from build123d import *

# Parameters (mm, degrees)
SKETCH1_W                           = 44
SKETCH1_H                           = 45
BASE_DEPTH                          = 5
WIRE_GROOVES_DEPTH                  = 51.338851795
SLANTED_START                       = -22
SLANTED_SCREW_PLATFORM_DEPTH        = 5
SKETCH5_R                           = 2.75
MOUNTING_HOLE_SCREW_INSERTION_DEPTH = 36.040152348
SKETCH6_W                           = 5
SKETCH6_H                           = 3
ZIP_TIE_SLOTS_DEPTH                 = 34.699235283
SKETCH7_R                           = 1.425
MOUNT_CLAMPING_HOLES_DEPTH          = 34.699235283
EDGE_FILLETS_R                      = 1


with BuildPart() as part:
    # Sketch1 → Base (new body)
    with BuildSketch(Plane.XY):
        Rectangle(SKETCH1_W, SKETCH1_H)
    extrude(amount=BASE_DEPTH)

    # Sketch2 → Wire Grooves (cut, through all)
    with BuildSketch(Plane(origin=(0, 22.5, 0), x_dir=(1, 0, 0), z_dir=(0, 1, 0))):
        with BuildLine():
            Line((12, 0), (18, 0))
            ThreePointArc((18, 0), (17.443502884, -1.343502884), (16.1, -1.9))
            Line((16.1, -1.9), (13.9, -1.9))
            ThreePointArc((13.9, -1.9), (12.556497116, -1.343502884), (12, 0))
        make_face()
        with BuildLine():
            Line((-7.7, -1.9), (-9.9, -1.9))
            ThreePointArc((-9.9, -1.9), (-11.243502884, -1.343502884), (-11.8, 0))
            Line((-11.8, 0), (-5.8, 0))
            ThreePointArc((-5.8, 0), (-6.356497116, -1.343502884), (-7.7, -1.9))
        make_face()
    extrude(amount=-WIRE_GROOVES_DEPTH, mode=Mode.SUBTRACT)

    # Sketch4 → Slanted Screw Platform (add, symmetric)
    with BuildSketch(Plane(origin=(22, 0, 0), x_dir=(0, 0, -1), z_dir=(1, 0, 0)).offset(SLANTED_START)):
        Polygon((-5, -22.5), (-5, 22.5), (-17.057713659, 22.5), align=None)
    extrude(amount=SLANTED_SCREW_PLATFORM_DEPTH, both=True)

    # Sketch5 → Mounting Hole Screw Insertion (cut, through all)
    with BuildSketch(Plane(origin=(0, -2.757214207, 10.290063509), x_dir=(1, 0, 0), z_dir=(0, -0.2588190451025216, 0.9659258262890681))):
        with Locations(Location((0, 16, 0), (0, 0, 270))):
            Circle(SKETCH5_R)
    extrude(amount=-MOUNTING_HOLE_SCREW_INSERTION_DEPTH, mode=Mode.SUBTRACT)

    # Sketch6 → Zip Tie Slots (cut, through all)
    with BuildSketch(Plane.XY.offset(5)):
        with Locations((-16, 18)):
            Rectangle(SKETCH6_W, SKETCH6_H)
        with Locations((8, 18)):
            Rectangle(SKETCH6_W, SKETCH6_H)
    extrude(amount=-ZIP_TIE_SLOTS_DEPTH, mode=Mode.SUBTRACT)

    # Sketch7 → Mount Clamping Holes (cut, through all)
    with BuildSketch(Plane.XY.offset(5)):
        with Locations((-18, -18.5)):
            Circle(SKETCH7_R)
        with Locations(Location((9, -18.5, 0), (0, 0, 180))):
            Circle(SKETCH7_R)
    extrude(amount=-MOUNT_CLAMPING_HOLES_DEPTH, mode=Mode.SUBTRACT)

    # Edge Fillets
    edge_fillets_edges = [part.edges().sort_by_distance(p)[0] for p in [
        (-22, 0, 5),
        (-13.5, 22.5, 5),
        (-5, 22.5, 11.02885683),
        (0, 22.5, 17.057713659),
        (22, 0, 5),
        (5, 22.5, 11.02885683),
        (22, -22.5, 2.5),
        (-22, -22.5, 2.5),
        (-22, 22.5, 2.5),
        (22, 22.5, 2.5),
        (13.5, 22.5, 5),
    ]]
    fillet(edge_fillets_edges, radius=EDGE_FILLETS_R)


solid = part.part
Check sheet for the modelled part. Datum: model origin and axes. Units: mm. A direction names the side the tool comes from. Give positions to 0.01 mm unless a question says otherwise; leave off trailing zeros. Loops run counter-clockwise (first coordinate to the right, second up) from the corner with the lowest first, then second, coordinate; pieces in that order, holes last. Notation, with made-up numbers: M 62,22 L 98,22 A23 ccw 98,58 Z; hole C 30,10.25 d7. An arc over 180 degrees is marked long. Use a Markdown table: item, result. Add a question column.
Q1. Sectioned sample at B-B, the plane y = -18.5. Record the cut outline in (x, z) (3 decimals), then the cut area to 3 significant figures.
Q2. Mould release check, pull along Y, two halves, no side actions. Record for faces 5 (the flat face through (-5, 5, 10)), 6 (the cylindrical face through (-12.381, 22.215, 4.699)), 7 (the flat face through (-18.5, 18, 3)), 8 (the flat face through (-16, 16.5, 3)): pulls with the +Y half, pulls with the -Y half, needs draft (parallel to the pull), parting line crosses it, or undercut.
Q3. Sectioned sample at C-C, the plane x = -2. Record the cut outline in (y, z), then the cut area to 3 significant figures.
Q4. Sectioned sample at D-D, the plane y = -6. Record the cut outline in (x, z).
Q5. Go/stop test with flat-tipped pins: pin 1 (1.1 mm diameter, centred on x = 15.5, y = -7.5, fed in from -Z); pin 2 (6 mm diameter, centred on y = 5.5, z = 13.5, fed in from +X); pin 3 (9.5 mm diameter, centred on y = 7.5, z = 11, fed in from -X); pin 4 (2.5 mm diameter, centred on x = 9, y = -18.5, fed in from +Z). Record where each tip stops, or that it passes through.
Q6. Scan lines: line 1 along Y through (x, z) = (-18, 3.4) (3 decimals); line 2 along Y through (x, z) = (9.5, 3.5); line 3 along X through (y, z) = (8, 6). Record each from-to range of solid material in increasing order. Write a range as [from, to].
Q7. Tool access check on faces 1 (the flat face through (5.5, 18, 3)), 2 (the cylindrical face through (-11.229, 0.315, 1.358)), 3 (the cylindrical face through (12.619, 22.215, 4.699)), 4 (the flat face through (-13, 0, 5)). Record the directions out of +Z, -Z, +X, -X, +Y, -Y that give a thin tool (end or side, any length) a straight path to the whole face; none if there is none.
Q8. Sectioned sample at A-A, the plane x = 9. Record the cut outline in (y, z) (3 decimals), then the cut area to 3 significant figures.
Verdict:
| question | item | result |
|---|---|---|
| 1 | outline | M -22,0 L -19.425,0 L -19.425,5 L -21,5 A1 ccw -22,4 Z; M -16.575,0 L -11.8,0 A1.9 cw -9.9,1.9 L -7.7,1.9 A1.9 cw -5.8,0 L 7.575,0 L 7.575,5 L 5,5 L 5,6.072 L -5,6.072 L -5,5 L -16.575,5 Z; M 10.425,0 L 12,0 A1.9 cw 13.9,1.9 L 16.1,1.9 A1.9 cw 18,0 L 22,0 L 22,4 A1 ccw 21,5 L 10.425,5 Z |
| 1 | area | 182 mm^2 |
| 2 | face 5 | needs draft |
| 2 | face 6 | pulls with the +Y half |
| 2 | face 7 | undercut |
| 2 | face 8 | undercut |
| 3 | outline | M -22.5,0 L 14.61,0 L 10.87,13.94 L -22.5,5 Z; M 14.52,14.92 L 18.52,0 L 22.5,0 L 22.5,15.75 A1 ccw 21.24,16.72 Z |
| 3 | area | 440 mm^2 |
| 4 | outline | M -22,0 L -11.8,0 A1.9 cw -9.9,1.9 L -7.7,1.9 A1.9 cw -5.8,0 L 12,0 A1.9 cw 13.9,1.9 L 16.1,1.9 A1.9 cw 18,0 L 22,0 L 22,4 A1 ccw 21,5 L 5,5 L 5,9.42 L -5,9.42 L -5,5 L -21,5 A1 ccw -22,4 Z |
| 5 | pin 1 | z = 1.9 |
| 5 | pin 2 | x = 5 |
| 5 | pin 3 | x = -5 |
| 5 | pin 4 | through |
| 6 | line 1 | [-22.5, -19.925], [-17.075, 16.5], [19.5, 22.5] |
| 6 | line 2 | [-22.5, -19.83], [-17.17, 16.5], [19.5, 22.5] |
| 6 | line 3 | [-5, 5] |
| 7 | face 1 | +Z, -Z |
| 7 | face 2 | -Z, +Y, -Y |
| 7 | face 3 | +Z, +X, +Y |
| 7 | face 4 | +Z, -X, +Y, -Y |
| 8 | outline | M -22.5,0 L -19.925,0 L -19.925,5 L -22.5,5 Z; M -17.075,0 L 16.5,0 L 16.5,5 L -17.075,5 Z; M 19.5,0 L 22.5,0 L 22.5,4 A1 ccw 21.5,5 L 19.5,5 Z |
| 8 | area | 196 mm^2 |
